```python
from build123d import *

# Parameters (mm, degrees)
F3_DEPTH        = 1.3
F3_COPIES_COUNT = 13


# Not quite as in the source:
# - a pattern or mirror of a feature is missing from the dataset's text; its kind, count and spacing are read off the source's solid


with BuildPart() as f1:
    # F0 (on Front) → F1 (revolve)
    with BuildSketch(Plane.XZ):
        Polygon((0, 3.4508320969), (0, 0), (10.5, 0), (10.5, 52), (8.5, 52), (8.5, 49.5), (7.1502993815, 49.5), (7.1502993815, 52), (0, 70.4032331705), (0, 44.7733812034), (7.0547335781, 44.7733812034), (7.0547335781, 3.4508320969), align=None)
    revolve(axis=Axis((0, 0, 35.2016165853), (0, 0, 1)))

    # F2 (on face) → F3 (cut)
    with BuildSketch(Plane.XY.offset(52)):
        with BuildLine():
            ThreePointArc((6.5231491988, 8.2279113103), (5.4797365468, 8.9567006971), (4.3558130739, 9.5538940995))
            Line((4.3558130739, 9.5538940995), (3.5032103316, 7.7445153091))
            ThreePointArc((3.5032103316, 7.7445153091), (4.4034584873, 7.2704575751), (5.2406151405, 6.6922307902))
            Line((5.2406151405, 6.6922307902), (6.5231491988, 8.2279113103))
        make_face()
    f3 = extrude(amount=-F3_DEPTH, mode=Mode.SUBTRACT)

    # F3_copies: F3 ×13 about axis
    f3_copies_axis = Axis((0, 0, 0), (0, 0, 1))
    for i in range(1, F3_COPIES_COUNT):
        add(f3.rotate(f3_copies_axis, i * 360 / F3_COPIES_COUNT), mode=Mode.SUBTRACT)


solid = f1.part
```
Design review of the part built by this model. Coordinates are the model's own, in mm. A direction names the side the tool comes from. Give positions to 0.01 mm unless a question says otherwise; leave off trailing zeros. Loops run counter-clockwise (first coordinate to the right, second up) from the corner with the lowest first, then second, coordinate; pieces in that order, holes last. Notation, with made-up numbers: (-20.75, -25.5) -> (-0.75, -25.5) arc R29 cw to (-0.75, 0.5) -> close; hole circle Ø2 at (-15, 52). An arc over 180 degrees is marked (long way). Write each question's results on one line, items separated by ' | '.
Q1. Machinability: for faces 1 (the face through (7.51, 5.84, 51.36)), 2 (the face through (8, 5, 50.7)), 3 (the face through (-8.69, -3.874, 51.359)), 4 (the face through (-9, 4, 52)), which of the approach directions +Z, -Z, +X, -X, +Y, -Y give a long, thin tool a straight path to every point of the face, cutting with its end or side? Answer none if there is none.
Reply:
face 1: +Z, +X | face 2: +Z | face 3: +Z, -X | face 4: +Z, -X, +Y, -Y
Q2. Wall thickness on L1, parallel to Y at x = 0, z = 51.2; L2, parallel to Y at x = 0, z = 31; L3, parallel to Z at x = -6.5, y = 5.25: over which ranges is each line inside the solid? List them lowest first.
Reply:
L1: y = -10.5 to -8.5, -7.15 to 7.15 | L2: y = -10.5 to -7.05, 7.05 to 10.5 | L3: z = 0 to 49.5
Q3. Take a section at A-A, the plane z = 64. Write out the cut boundary in (x, y).
Reply:
outline: circle Ø4.98 at (0, 0)
Q4. The part is to be moulded in two halves that separate along Y. For faces 5 (the face through (-0.54, 9.5, 51.36)), 6 (the face through (9.36, 1.68, 51.36)), 7 (the face through (7, -6, 52)), 8 (the face through (-3.9, -8.6, 51.4)), say which applies: +Y half, -Y half, draft (parallel to the pull), parting line (faces both ways), or undercut.
Reply:
face 5: +Y half | face 6: undercut | face 7: draft | face 8: -Y half
Q5. For pin 1 Ø3.5 at (x, y) = (-6.5, -7.5) entering from +Z; pin 2 Ø5 at (y, z) = (-5.5, 17.5) entering from +X; pin 3 Ø1.4 at (x, y) = (-4.5, 9.5) entering from +Z; pin 4 Ø6 at (x, z) = (3, 38) entering from +Y, all flat-tipped, find the tip position at first contact; note any pin that passes through.
Reply:
pin 1: stops at z = 52 | pin 2: stops at x = 10.06 | pin 3: stops at z = 50.7 | pin 4: stops at y = 10.5
